Autodesk Inventor part; units mm, degrees
ref_plane "YZ Plane" through (0, 0, 0) normal (1, 0, 0) x (0, 1, 0)
ref_plane "XZ Plane" through (0, 0, 0) normal (0, 1, 0) x (-1, 0, 0)
ref_plane "XY Plane" through (0, 0, 0) normal (0, 0, 1) x (1, 0, 0)
sketch "Sketch1" plane through (0, 0, 0) normal (1, 0, 0) x (0, 1, 0)
  line L0 (25.4, 25.4) -> (-25.4, 25.4)
  line L1 (-25.4, 25.4) -> (-25.4, -25.4)
  line L2 (-25.4, -25.4) -> (25.4, -25.4)
  line L3 (25.4, -25.4) -> (25.4, 25.4)
  line L4 (23.2918, 23.2918) -> (-23.2918, 23.2918)
  line L5 (-23.2918, 23.2918) -> (-23.2918, -23.2918)
  line L6 (-23.2918, -23.2918) -> (23.2918, -23.2918)
  line L7 (23.2918, -23.2918) -> (23.2918, 23.2918)
  point P0 (0, 0)
  point P1 (0, -25.4)
  point P2 (25.4, 0)
  dimension "d0" = 50.8
  dimension "d1" = 50.8
  dimension "d2" = 2.1082
extrude "Extrusion1" add sketch "Sketch1" along normal blind 304.8
fillet "Fillet1" radius 3.175 4 edges at (152.4, 25.4, 25.4) (152.4, -25.4, 25.4) (152.4, 25.4, -25.4) (152.4, -25.4, -25.4)
sketch "Sketch2" plane through (0, -22.225, 25.4) normal (0, 0, 1) x (1, 0, 0)
  line L0 (0, 44.45) -> (0, 0)
  line L1 (304.8, 44.45) -> (304.8, 0)
  line L2 (0, -3.175) -> (0, 47.625)
  line L3 (0, 45.5168) -> (0, -1.0668)
  line L4 (0, 47.625) -> (50.8, -3.175)
  line L5 (0, -3.175) -> (50.8, -3.175)
  line L6 (304.8, -3.175) -> (304.8, 47.625)
  line L7 (304.8, 47.625) -> (254, -3.175)
  line L8 (254, -3.175) -> (304.8, -3.175)
  line L9 (0, -3.175) -> (304.8, -3.175)
  point P0 (0, 22.225)
  dimension "d6" = 45
  dimension "d7" = 45
extrude "Extrusion2" cut sketch "Sketch2" against normal through all
properties part number "45degree_brace" material "Steel"
For this review, take the finished solid that the model builds, in its own axes (mm). A direction names the side the tool comes from. Give positions to 0.01 mm unless a question says otherwise; leave off trailing zeros. Write each loop counter-clockwise with the first axis right and the second up, starting at its lowest first coordinate (ties: lowest second). Pieces come first, ordered by that corner, then holes. Notation, with made-up numbers: (-35, 56.25) -> (17, 56.25) arc R12 cw to (17, 64.25) -> close; hole circle Ø8 at (-16, 50). An arc over 180 degrees is marked (long way). Use CSV: the item, a comma, the result in double quotes.
Q1. Take a section at C-C, the plane z = 9. Write out the cut boundary in (x, y).
Conclusion:
outline,"(0, 25.4) -> (2.11, 23.29) -> (302.69, 23.29) -> (304.8, 25.4) -> close; (48.69, -23.29) -> (50.8, -25.4) -> (254, -25.4) -> (256.11, -23.29) -> close"
Q2. Take a section at B-B, the plane x = 107. Write out the cut boundary in (y, z) (3 decimals).
Conclusion:
outline,"(-25.4, -22.225) arc R3.175 ccw to (-22.225, -25.4) -> (22.225, -25.4) arc R3.175 ccw to (25.4, -22.225) -> (25.4, 22.225) arc R3.175 ccw to (22.225, 25.4) -> (-22.225, 25.4) arc R3.175 ccw to (-25.4, 22.225) -> close; hole (-23.292, -23.292) -> (23.292, -23.292) -> (23.292, 23.292) -> (-23.292, 23.292) -> close"
Q3. Mouldability with a two-part tool opening along Z and no side actions: class faces 1 (the face through (150, 0, -23.292)), 2 (the face through (150, 0, 25.4)), 3 (the face through (279.5, 0.1, -24.3)), 4 (the face through (151, -23.292, 0)) as pulls with the +Z half, pulls with the -Z half, needs draft (parallel to the pull), parting line crosses it, or undercut.
Conclusion:
face 1,"undercut"
face 2,"pulls with the +Z half"
face 3,"needs draft"
face 4,"undercut"
Q4. To check wall thickness, follow probe 1 along Z at (x, y) = (224, 20); probe 2 along Y at (x, z) = (49, 12). State the ranges of each line that lie inside material, in increasing order. Write a range as [from, to].
Conclusion:
probe 1,"[-25.4, -23.29], [23.29, 25.4]"
probe 2,"[-23.6, -23.29], [23.29, 25.4]"
Q5. Tool access review of faces 5 (the face through (150, 25.4, 0)), 6 (the face through (150, 23.292, 0)): name each direction out of +Z, -Z, +X, -X, +Y, -Y from which nothing blocks a thin tool from reaching the whole face with its end or side.
Conclusion:
face 5,"+Z, -Z, +X, -X, +Y"
face 6,"+X, -X"
Q6. Take a section at A-A, the plane y = 4. Write out the cut boundary in (x, z).
Conclusion:
outline,"(21.4, -25.4) -> (283.4, -25.4) -> (283.4, -23.29) -> (21.4, -23.29) -> close; (21.4, 23.29) -> (283.4, 23.29) -> (283.4, 25.4) -> (21.4, 25.4) -> close"
